```python
from build123d import *

# Parameters (mm, degrees)
SKETCH1_R           = 40
SKETCH1_R_2         = 35
BOSS_EXTRUDE1_DEPTH = 10
CUT_EXTRUDE5_DEPTH  = 10
CIRPATTERN2_COUNT   = 30


with BuildPart() as part:
    # Sketch1 → Boss-Extrude1 (new body)
    with BuildSketch(Plane.XY):
        Circle(SKETCH1_R)
        Circle(SKETCH1_R_2, mode=Mode.SUBTRACT)
    extrude(amount=BOSS_EXTRUDE1_DEPTH)

    # Sketch4 → Cut-Extrude5 (cut)
    with BuildSketch(Plane.XY):
        with BuildLine():
            Line((2, 37.947331922), (2, 39.949968711))
            ThreePointArc((2, 39.949968711), (0, 40), (-2, 39.949968711))
            Line((-2, 39.949968711), (-2, 37.947331922))
            ThreePointArc((-2, 37.947331922), (0, 38), (2, 37.947331922))
        make_face()
    cut_extrude5 = extrude(amount=CUT_EXTRUDE5_DEPTH, mode=Mode.SUBTRACT)

    # CirPattern2: Cut-Extrude5 ×30 about axis
    cirpattern2_axis = Axis((0, 0, 0), (0, 0, 1))
    for i in range(1, CIRPATTERN2_COUNT):
        add(cut_extrude5.rotate(cirpattern2_axis, i * 360 / CIRPATTERN2_COUNT), mode=Mode.SUBTRACT)


solid = part.part
```
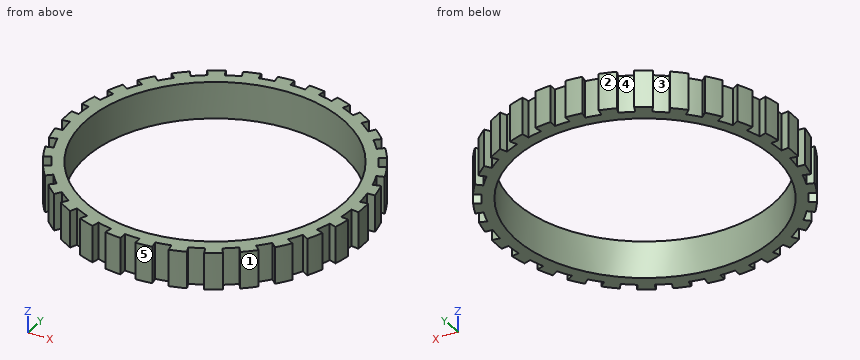
Work out the finished part from the listing and answer in its coordinate system (mm). Face numbers are marked on the shaded views. A direction names the side the tool comes from. Coordinates: 2 decimals unless noted, no trailing zeros. Loops run counter-clockwise (first coordinate to the right, second up) from the corner with the lowest first, then second, coordinate; pieces in that order, holes last. Notation, with made-up numbers: M 22,7.5 L 67,7.5 A28 cw 67,34.5 Z; hole C 44,-21.5 d9. An arc over 180 degrees is marked long. Use CSV: the item, a comma, the result in double quotes. Start each with the question number.
(1) Consider line 1 (Y direction, x = 1, z = 7); line 2 (Y direction, x = 5, z = 2); line 3 (X direction, y = -27, z = 0.75). Determine where each line is inside the solid, lowest interval first.
(2) Given pin 1 Ø5 at (x, z) = (20, 7) entering from -Y; pin 2 Ø5 at (x, z) = (8.5, 7) entering from -Y; pin 3 Ø2 at (x, y) = (22.5, 26) entering from +Z; pin 4 Ø2 at (x, z) = (-26.5, 2.5) entering from +Y, each flat-ended and moving along its own axis, determine where each tip first touches the part or whether it passes through.
(3) Find section A-A, the plane y = 0. Give the vertices of the cut face in (x, z).
(4) For a pull along X with two mould halves and no side action, classify the marked faces 1, 2 and 3 as +X half, -X half, draft (parallel to the pull), parting line (faces both ways), or undercut.
(5) Find section B-B, the plane x = 0. Give the vertices of the cut face in (y, z), then the cut area to 3 significant figures.
(6) For the marked faces 4 and 5, determine the directions among +Z, -Z, +X, -X, +Y, -Y from which every point of the face is accessible in a straight line to the end or side of a thin tool.
Recorded:
1,line 1,"y = -37.99 to -34.99, 34.99 to 37.99"
1,line 2,"y = -39.69 to -34.64, 34.64 to 39.69"
1,line 3,"x = -27 to -22.27, 22.27 to 27"
2,pin 1,"stops at y = -35.68"
2,pin 2,"stops at y = -39.55"
2,pin 3,"stops at z = 10"
2,pin 4,"stops at y = 30.82"
3,outline,"M -40,0 L -35,0 L -35,10 L -40,10 Z; M 35,0 L 40,0 L 40,10 L 35,10 Z"
4,face 1,"+X half"
4,face 2,"-X half"
4,face 3,"undercut"
5,outline,"M -38,0 L -35,0 L -35,10 L -38,10 Z; M 35,0 L 38,0 L 38,10 L 35,10 Z"
5,area,"60.0 mm^2"
6,face 4,"+Z, -Z"
6,face 5,"+Z, -Z, +X, -Y"
